```python
from build123d import *

# Parameters (mm, degrees)
P_IDAT_VYSUNUT_M2_REACH = 502
SKICA2_W                = 35
SKICA2_H                = 250


with BuildPart() as part:
    # Skica1 → Rotovat1 (revolve)
    with BuildSketch(Plane.XY):
        with BuildLine():
            Line((200, 200), (800, 200))
            ThreePointArc((800, 200), (941.421356237, 141.421356237), (1000, 0))
            Line((1000, 0), (990, 0))
            ThreePointArc((990, 0), (934.350288425, 134.350288425), (800, 190))
            Line((800, 190), (200, 190))
            ThreePointArc((200, 190), (65.649711575, 134.350288425), (10, 0))
            Line((10, 0), (0, 0))
            ThreePointArc((0, 0), (58.578643763, 141.421356237), (200, 200))
        make_face()
    revolve(axis=Axis((0, 0, 0), (1, 0, 0)))

    # Skica2 → Přidat vysunutím2 (add, up to next)
    with BuildSketch(Plane.XY.offset(300), mode=Mode.PRIVATE) as p_idat_vysunut_m2_sk1:
        with Locations((717.5, 0)):
            Rectangle(SKICA2_W, SKICA2_H)
    p_idat_vysunut_m2_tool1 = extrude(p_idat_vysunut_m2_sk1.sketch, amount=-P_IDAT_VYSUNUT_M2_REACH, mode=Mode.PRIVATE) - part.part
    add(p_idat_vysunut_m2_tool1.solids().sort_by_distance((717.5, 0, 300))[0])
    # Skica2 → Přidat vysunutím2 (add, up to next)
    with BuildSketch(Plane.XY.offset(300), mode=Mode.PRIVATE) as p_idat_vysunut_m2_sk2:
        with Locations((282.5, 0)):
            Rectangle(SKICA2_W, SKICA2_H)
    p_idat_vysunut_m2_tool2 = extrude(p_idat_vysunut_m2_sk2.sketch, amount=-P_IDAT_VYSUNUT_M2_REACH, mode=Mode.PRIVATE) - part.part
    add(p_idat_vysunut_m2_tool2.solids().sort_by_distance((282.5, 0, 300))[0])


solid = part.part
```
Geometry check sheet. Reference: the model listing, model coordinates, mm. A direction names the side the tool comes from. Coordinates: 2 decimals unless noted, no trailing zeros. Loops run counter-clockwise (first coordinate to the right, second up) from the corner with the lowest first, then second, coordinate; pieces in that order, holes last.
Item 1: Thickness scan on line 1 (Z direction, x = 479, y = 0); line 2 (X direction, y = 73, z = 252); line 3 (Z direction, x = 664, y = 99). Record the ranges inside material, lowest first.
Item 2: Sectioned sample at B-B, the plane y = 0. Record the boundary of the cut face in (x, z), then the cut area to 3 significant figures.
Item 3: Go/stop test with flat-tipped pins: pin 1 Ø3 at (x, z) = (260, -66) entering from -Y; pin 2 Ø10 at (y, z) = (-1, 29) entering from -X; pin 3 Ø12 at (x, z) = (504, 153) entering from -Y. Record where each tip stops, or that it passes through.
Item 4: Release check for a two-part mould opening along X. For faces 5 (the face through (735, -2, 245)), 6 (the face through (504.2, -43.356, -195.244)), 7 (the face through (717, 2, 300)) record: released by +X, released by -X, zero draft, split by the parting line, or undercut.
Item 5: Sectioned sample at D-D, the plane x = 690. Record the boundary of the cut face in (y, z), then the cut area to 3 significant figures.
Item 6: Sectioned sample at C-C, the plane z = 0. Record the boundary of the cut face in (x, y), then the cut area to 3 significant figures.
Item 7: Access from +Z, -Z, +X, -X, +Y, -Y to the whole of each face (thin tool, end or side, straight path). Record for faces 1 (the face through (282, 2, 300)), 2 (the face through (495.8, -41.19, -185.48)), 3 (the face through (282, 125, 229)), 4 (the face through (717, -125, 229)).
Item 8: Sectioned sample at A-A, the plane z = 231. Record the boundary of the cut face in (x, y).
Check result:
1. line 1: z = -200 to -190, 190 to 200
1. line 2: x = 265 to 300, 700 to 735
1. line 3: z = -173.78 to -162.17, 162.17 to 173.78
2. outline: (200, -200) - (800, -200) arc R200 ccw to (800, 200) - (735, 200) - (735, 300) - (700, 300) - (700, 200) - (300, 200) - (300, 300) - (265, 300) - (265, 200) - (200, 200) arc R200 ccw to start; hole (200, -190) - (800, -190) arc R190 ccw to (800, 190) - (200, 190) arc R190 ccw to start
2. area: 31,300 mm2
3. pin 1: stops at y = -189.31
3. pin 2: stops at x = 1.45
3. pin 3: stops at y = -135.61
4. face 5: released by +X
4. face 6: undercut
4. face 7: zero draft
5. outline: circle Ø400 at (0, 0); hole circle Ø380 at (0, 0)
5. area: 12,300 mm2
6. outline: (200, -200) - (800, -200) arc R200 ccw to (800, 200) - (200, 200) arc R200 ccw to start; hole (200, -190) - (800, -190) arc R190 ccw to (800, 190) - (200, 190) arc R190 ccw to start
6. area: 24,300 mm2
7. face 1: +Z, +X, -X, +Y, -Y
7. face 2: none
7. face 3: +Z, +X, -X, +Y
7. face 4: +Z, +X, -X, -Y
8. outline: (265, -125) - (300, -125) - (300, 125) - (265, 125) - close; (700, -125) - (735, -125) - (735, 125) - (700, 125) - close
